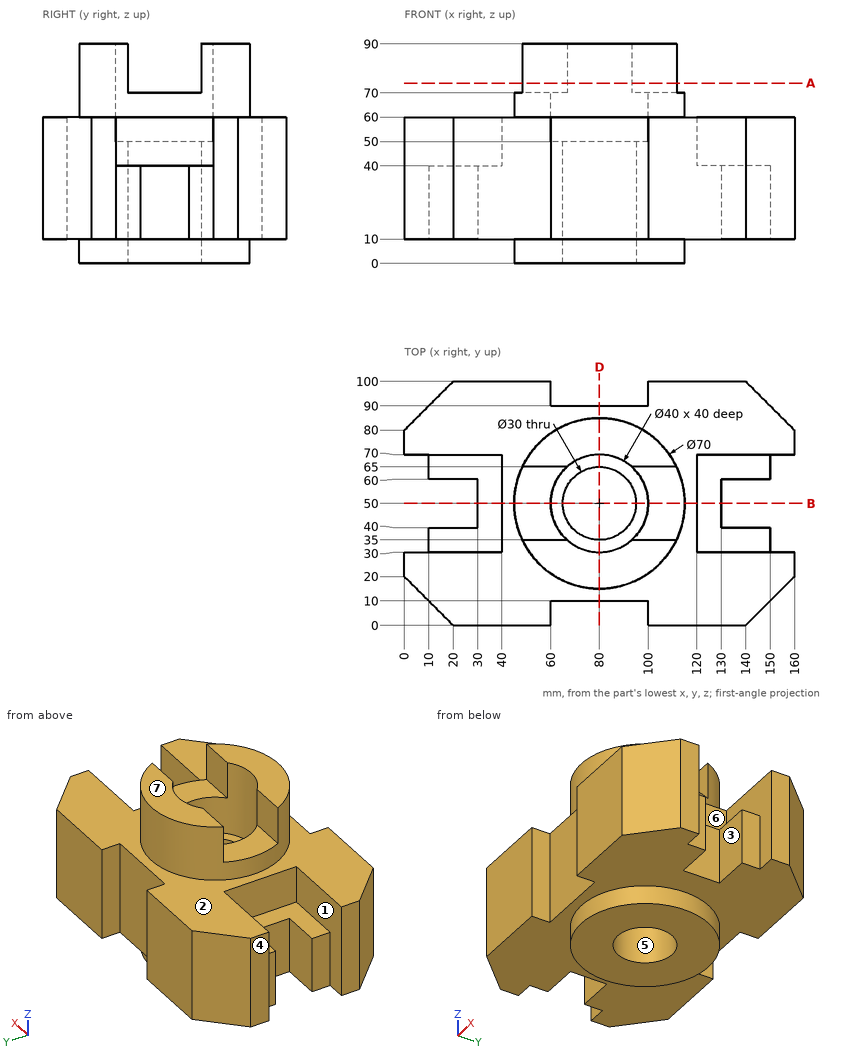
Print and shaded views of the part. All mm, measured from the part's lowest x, y and z. A direction names the side the tool comes from. Coordinates: 2 decimals unless noted, no trailing zeros. Order: outer loops, then holes, each group sorted by start corner. A loop starts at its lowest first (then second) coordinate and runs counter-clockwise, first axis right, second up.
(1) Slice it at B-B, the plane y = 50. Write the cut outline in (x, z).
Check sheet entries:
outline: (30, 10) - (45, 10) - (45, 0) - (65, 0) - (65, 50) - (60, 50) - (60, 70) - (45, 70) - (45, 60) - (40, 60) - (40, 40) - (30, 40) - close; (95, 0) - (115, 0) - (115, 10) - (130, 10) - (130, 40) - (120, 40) - (120, 60) - (115, 60) - (115, 70) - (100, 70) - (100, 50) - (95, 50) - close
(2) Slice it at A-A, the plane z = 74. Write the cut outline in (x, y).
Check sheet entries:
outline: (48.38, 35) arc R35 ccw to (111.62, 35) - (93.23, 35) arc R20 cw to (66.77, 35) - close; (48.38, 65) - (66.77, 65) arc R20 cw to (93.23, 65) - (111.62, 65) arc R35 ccw to start
(3) Pull direction X, two halves, no side cores. Call the marked faces 4, 5, 6 and 7: pulls with the +X half, pulls with the -X half, needs draft (parallel to the pull), parting line crosses it, or undercut.
Check sheet entries:
face 4: pulls with the -X half
face 5: undercut
face 6: pulls with the +X half
face 7: needs draft
(4) Pin check, flat tips, straight feed: pin 1 Ø10 at (x, z) = (73.5, 79) entering from -Y; pin 2 Ø1.5 at (y, z) = (57.5, 9) entering from -X; pin 3 Ø22 at (y, z) = (57.5, 46.5) entering from -X. Stop position of each tip, or through.
Check sheet entries:
pin 1: stops at y = 15.03
pin 2: stops at x = 45.66
pin 3: stops at x = 10
(5) Probe L1, parallel to Y at x = 80, z = 11; L2, parallel to Y at x = 80, z = 72; L3, parallel to Z at x = 119, y = 73.5. List the from-to ranges inside material, lowest first.
Check sheet entries:
L1: y = 10 to 35, 65 to 90
L2: y = 15 to 30, 70 to 85
L3: z = 10 to 60
(6) Tool access for the marked faces 1, 2 and 3: list every direction of +Z, -Z, +X, -X, +Y, -Y with a clear straight run to the whole face (end or side of a thin tool).
Check sheet entries:
face 1: +Z, -X
face 2: +Z
face 3: +Z, -Z, +X
(7) Slice it at D-D, the plane x = 80. Write the cut outline in (y, z).
Check sheet entries:
outline: (10, 10) - (15, 10) - (15, 0) - (35, 0) - (35, 50) - (30, 50) - (30, 90) - (15, 90) - (15, 60) - (10, 60) - close; (65, 0) - (85, 0) - (85, 10) - (90, 10) - (90, 60) - (85, 60) - (85, 90) - (70, 90) - (70, 50) - (65, 50) - close
